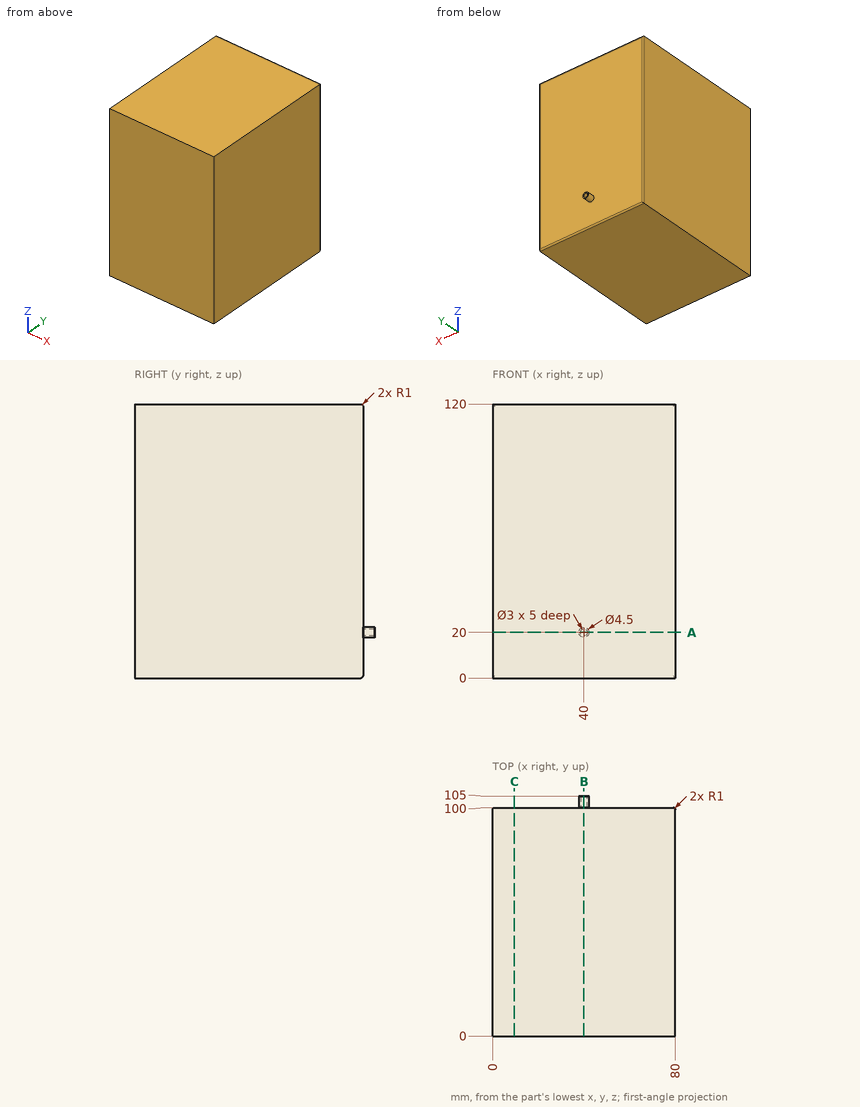
Design review of the part shown in the three views and the two pictorial views. Dimensions are in mm from the part's minimum x, y and z. Coordinates: 2 decimals unless noted, no trailing zeros. Loops run counter-clockwise (first coordinate to the right, second up) from the corner with the lowest first, then second, coordinate; pieces in that order, holes last. Notation, with made-up numbers: M 56.5,84.5 L 67.5,84.5 A18 ccw 67.5,105.5 Z; hole C 28,-38 d4. An arc over 180 degrees is marked long. Put each result on its own line as item: value. Start each with the question number.
Q1. Clearance check with flat-ended pins moving along their axes: pin 1 (23.5 mm diameter, centred on x = 42.5, z = 78, fed in from +Y); pin 2 (1 mm diameter, centred on x = 11.5, z = 58.5, fed in from -Y). State where each tip first meets the part, or that it passes through.
Q2. Add section C-C (x = 9.5). Write out the cut boundary in (y, z), and give its area (3 significant figures).
Q3. Wall thickness on line 1 (Z direction, x = 40, y = 101); line 2 (X direction, y = 102.9, z = 20); line 3 (Y direction, x = 26, z = 82): over which ranges is each line inside the solid? List them lowest first.
Q4. Add section A-A (z = 20). Write out the cut boundary in (x, y).
Q5. Add section B-B (x = 40). Write out the cut boundary in (y, z), and give its area (3 significant figures).
Answers:
1. pin 1: stops at y = 100
1. pin 2: stops at y = 0
2. outline: M 0,0 L 99,0 A1 ccw 100,1 L 100,119 A1 ccw 99,120 L 0,120 Z
2. area: 12,000 mm^2
3. line 1: z = 17.75 to 18.5, 21.5 to 22.25
3. line 2: x = 37.75 to 38.5, 41.5 to 42.25
3. line 3: y = 0 to 100
4. outline: M 0,0 L 80,0 L 80,99 A1 ccw 79,100 L 42.25,100 L 42.25,105 L 41.5,105 L 41.5,100 L 38.5,100 L 38.5,105 L 37.75,105 L 37.75,100 L 1,100 A1 ccw 0,99 Z
5. outline: M 0,0 L 99,0 A1 ccw 100,1 L 100,17.75 L 105,17.75 L 105,18.5 L 100,18.5 L 100,21.5 L 105,21.5 L 105,22.25 L 100,22.25 L 100,119 A1 ccw 99,120 L 0,120 Z
5. area: 12,000 mm^2
